Source: CAD feature listing. Evaluate the final solid. Frame: model axes, mm. Face numbers are marked on the shaded views. A direction names the side the tool comes from. Coordinates: 2 decimals unless noted, no trailing zeros. Write each loop counter-clockwise with the first axis right and the second up, starting at its lowest first coordinate (ties: lowest second). Pieces come first, ordered by that corner, then holes. Notation, with made-up numbers: M 62.25,-20.75 L 69.25,-20.75 A15 cw 69.25,6.25 Z; hole C 55.25,45.25 d1. An arc over 180 degrees is marked long. Answer as CSV lines item,"result". Start each with the question number.
1. Contact query for flat-ended pins moving along their axis: pin 1 Ø1.5 at (y, z) = (2.5, 8) entering from -X; pin 2 Ø4 at (x, y) = (-12.5, -1) entering from +Z; pin 3 Ø1.2 at (y, z) = (0, 2) entering from -X. Output: stop coordinate, or through.
2. Section A-A on y = 9. Return the cut outline in (x, z).
3. Reachability of the marked faces 1, 2, 3 and 4 from +Z, -Z, +X, -X, +Y, -Y: full face, straight path, thin tool, end or side. Return the list, or none.
4. Mould query, pull axis Y, two halves, no side actions, for the marked faces 5, 6, 7 and 8. Classes: pulls with the +Y half, pulls with the -Y half, needs draft (parallel to the pull), parting line crosses it, or undercut.
5. Line query: probe 1 along Y at (x, z) = (-13.25, 0); probe 2 along Y at (x, z) = (-8.25, -1); probe 3 along X at (y, z) = (7.25, -8.75). Output: solid intervals per line, ascending. Write a range as [from, to].
6. Section D-D on x = -14. Return the cut outline in (y, z).
7. Section C-C on x = -7.5. Return the cut outline in (y, z).
8. Section B-B on z = 0. Return the cut outline in (x, y), plus the area to 3 significant figures.
```python
from build123d import *

# Parameters (mm, degrees)
BODY1_DEPTH    = 5
BODY2_SKETCH_W = 8
BODY2_SKETCH_H = 24
BODY2_DEPTH    = 10
CUT_SKETCH_R   = 2.5
CUT_DEPTH      = 10
SKETCH2_W      = 9.7
SKETCH2_H      = 12
L_DETAIL_DEPTH = 24


with BuildPart() as part:
    # Body1_Sketch → Body1 (new body, symmetric)
    with BuildSketch(Plane.XY):
        Polygon((-16.5, -12), (-16.5, -2), (-14.5, -2), (-14.5, 2), (-16.5, 2), (-16.5, 12), (0, 12), (0, -12), align=None)
    extrude(amount=BODY1_DEPTH, both=True)

    # Body2_Sketch → Body2 (add, symmetric)
    with BuildSketch(Plane.XY):
        with Locations((-4, 0)):
            Rectangle(BODY2_SKETCH_W, BODY2_SKETCH_H)
    extrude(amount=BODY2_DEPTH, both=True)

    # Cut_Sketch → Cut (cut)
    with BuildSketch(Plane.ZY.offset(16.5)):
        with Locations((0, 7)):
            Circle(CUT_SKETCH_R)
        with Locations((0, -7)):
            Circle(CUT_SKETCH_R)
    extrude(amount=-CUT_DEPTH, mode=Mode.SUBTRACT)

    # Sketch2 → L-Detail (add)
    with BuildSketch(Plane(origin=(0, 12, 0), x_dir=(-1, 0, 0), z_dir=(0, 1, 0))):
        with Locations((-4.85, 0)):
            Rectangle(SKETCH2_W, SKETCH2_H)
    extrude(amount=-L_DETAIL_DEPTH)


solid = part.part
```
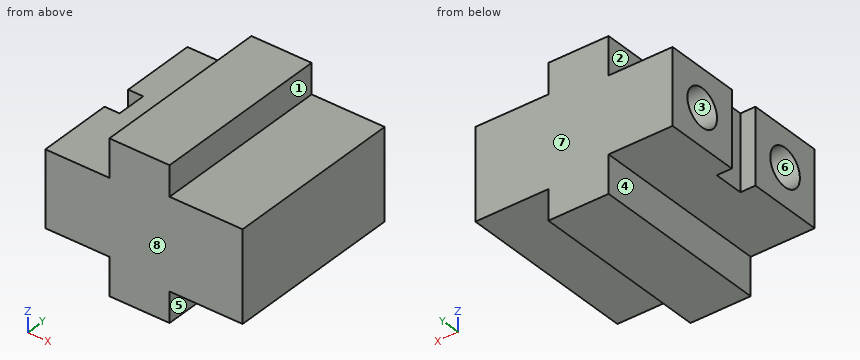
Values:
1,pin 1,"x = -8"
1,pin 2,"z = 5"
1,pin 3,"x = -14.5"
2,outline,"M -16.5,-5 L -8,-5 L -8,-10 L 0,-10 L 0,-6 L 9.7,-6 L 9.7,6 L 0,6 L 0,10 L -8,10 L -8,5 L -16.5,5 L -16.5,1.5 L -6.5,1.5 L -6.5,-1.5 L -16.5,-1.5 Z"
3,face 1,"+Z, +X, +Y, -Y"
3,face 2,"+Z, -X, +Y, -Y"
3,face 3,"-X"
3,face 4,"-Z, -X, +Y, -Y"
4,face 5,"needs draft"
4,face 6,"undercut"
4,face 7,"pulls with the +Y half"
4,face 8,"pulls with the -Y half"
5,probe 1,"[-12, -9.5], [-4.5, 4.5], [9.5, 12]"
5,probe 2,"[-12, -9.29], [-4.71, 4.71], [9.29, 12]"
5,probe 3,"[-8, 0]"
6,outline,"M -12,-5 L 12,-5 L 12,5 L -12,5 Z; hole C -7,0 d5; hole C 7,0 d5"
7,outline,"M -12,-10 L 12,-10 L 12,10 L -12,10 Z; hole C -7,0 d5; hole C 7,0 d5"
8,outline,"M -16.5,-12 L 9.7,-12 L 9.7,12 L -16.5,12 L -16.5,9.5 L -6.5,9.5 L -6.5,4.5 L -16.5,4.5 L -16.5,2 L -14.5,2 L -14.5,-2 L -16.5,-2 L -16.5,-4.5 L -6.5,-4.5 L -6.5,-9.5 L -16.5,-9.5 Z"
8,area,"521 mm²"
